from build123d import *

# Parameters (mm, degrees)
SKETCH1_W             = 278.511
SKETCH1_H             = 129.9972
BOSS_EXTRUDE1_DEPTH   = 4.191
F_2_56_TAPPED_HOLE2_D = 1.778
F_8_32_TAPPED_HOLE1_D = 3.4544
CUT_EXTRUDE1_REACH    = 309.384
SKETCH25_R            = 22.86
CUT_EXTRUDE2_REACH    = 309.384
SKETCH27_R            = 4.1656
SKETCH27_R_2          = 1.905


with BuildPart() as part:
    # Sketch1 → Boss-Extrude1 (new body)
    with BuildSketch(Plane(origin=(0, 0, 0), x_dir=(0, 0, -1), z_dir=(1, 0, 0))):
        with Locations((139.2555, 64.9986)):
            Rectangle(SKETCH1_W, SKETCH1_H)
    extrude(amount=BOSS_EXTRUDE1_DEPTH)

    # #2-56 Tapped Hole2 (through all)
    with Locations(Plane(origin=(4.191, 0, 0), x_dir=(0, 0, -1), z_dir=(1, 0, 0))):
        with Locations((38.1, 83.9724), (38.1, 110.9472), (60.452, 97.4598), (73.152, 110.9472), (73.152, 83.9724), (95.504, 97.4598)):
            Hole(F_2_56_TAPPED_HOLE2_D / 2)

    # #8-32 Tapped Hole1 (through all)
    with Locations(Plane(origin=(4.191, 0, 0), x_dir=(0, 0, -1), z_dir=(1, 0, 0))):
        with Locations((114.3, 60.9092), (114.3, 110.9472), (164.338, 110.9472), (164.338, 60.9092)):
            Hole(F_8_32_TAPPED_HOLE1_D / 2)

    # Sketch25 → Cut-Extrude1 (cut, up to next)
    with BuildSketch(Plane(origin=(4.191, 0, 0), x_dir=(0, 0, -1), z_dir=(1, 0, 0)), mode=Mode.PRIVATE) as cut_extrude1_sk1:
        with Locations((139.319, 85.9282)):
            Circle(SKETCH25_R)
    cut_extrude1_tool1 = extrude(cut_extrude1_sk1.sketch, amount=-CUT_EXTRUDE1_REACH, mode=Mode.PRIVATE) & part.part
    add(cut_extrude1_tool1.solids().sort_by_distance((4.191, 85.9282, -139.319))[0], mode=Mode.SUBTRACT)

    # Sketch27 → Cut-Extrude2 (cut, up to next)
    with BuildSketch(Plane(origin=(4.191, 0, 0), x_dir=(0, 0, -1), z_dir=(1, 0, 0)), mode=Mode.PRIVATE) as cut_extrude2_sk1:
        with Locations((221.361, 98.2472)):
            Circle(SKETCH27_R)
    cut_extrude2_tool1 = extrude(cut_extrude2_sk1.sketch, amount=-CUT_EXTRUDE2_REACH, mode=Mode.PRIVATE) & part.part
    # Sketch27 → Cut-Extrude2 (cut, up to next)
    with BuildSketch(Plane(origin=(4.191, 0, 0), x_dir=(0, 0, -1), z_dir=(1, 0, 0)), mode=Mode.PRIVATE) as cut_extrude2_sk2:
        with Locations((211.836, 98.2472)):
            Circle(SKETCH27_R_2)
    cut_extrude2_tool2 = extrude(cut_extrude2_sk2.sketch, amount=-CUT_EXTRUDE2_REACH, mode=Mode.PRIVATE) & part.part
    # Sketch27 → Cut-Extrude2 (cut, up to next)
    with BuildSketch(Plane(origin=(4.191, 0, 0), x_dir=(0, 0, -1), z_dir=(1, 0, 0)), mode=Mode.PRIVATE) as cut_extrude2_sk3:
        with Locations((230.886, 98.2472)):
            Circle(SKETCH27_R)
    cut_extrude2_tool3 = extrude(cut_extrude2_sk3.sketch, amount=-CUT_EXTRUDE2_REACH, mode=Mode.PRIVATE) & part.part
    # Sketch27 → Cut-Extrude2 (cut, up to next)
    with BuildSketch(Plane(origin=(4.191, 0, 0), x_dir=(0, 0, -1), z_dir=(1, 0, 0)), mode=Mode.PRIVATE) as cut_extrude2_sk4:
        with Locations((240.411, 98.2472)):
            Circle(SKETCH27_R_2)
    cut_extrude2_tool4 = extrude(cut_extrude2_sk4.sketch, amount=-CUT_EXTRUDE2_REACH, mode=Mode.PRIVATE) & part.part
    add(cut_extrude2_tool1.solids().sort_by_distance((4.191, 98.2472, -221.361))[0], mode=Mode.SUBTRACT)
    add(cut_extrude2_tool2.solids().sort_by_distance((4.191, 98.2472, -211.836))[0], mode=Mode.SUBTRACT)
    add(cut_extrude2_tool3.solids().sort_by_distance((4.191, 98.2472, -230.886))[0], mode=Mode.SUBTRACT)
    add(cut_extrude2_tool4.solids().sort_by_distance((4.191, 98.2472, -240.411))[0], mode=Mode.SUBTRACT)


solid = part.part
Could you check a few things on this model? Use its own coordinates, in mm. Round coordinates to 2 decimals unless told otherwise and drop trailing zeros. Loops run counter-clockwise (first coordinate to the right, second up) from the corner with the lowest first, then second, coordinate; pieces in that order, holes last. Notation, with made-up numbers: (25.5, 50.25) -> (47.5, 50.25) arc R37 cw to (47.5, 86.25) -> close; hole circle Ø7 at (46, 3.5). An arc over 180 degrees is marked (long way). Use CSV: the item, a comma, the result in double quotes.
(1) Suppose I cut it at A-A on y = 74. Write out the boundary of the cut face in (x, z).
Return value:
outline,"(0, -278.51) -> (4.19, -278.51) -> (4.19, -158.82) -> (0, -158.82) -> close; (0, -119.82) -> (4.19, -119.82) -> (4.19, 0) -> (0, 0) -> close"
(2) If I drill on probe 1 along Y at (x, z) = (0.9, -38.1); probe 2 along Z at (x, y) = (3.95, 111); probe 3 along Z at (x, y) = (1.55, 99), over which ranges is the centre line in solid material (lowest first)? Write a range as [from, to].
Return value:
probe 1,"y = [0, 83.08], [84.86, 110.06], [111.84, 130]"
probe 2,"z = [-278.51, -166.06], [-162.61, -116.03], [-112.57, -74.04], [-72.26, -38.99], [-37.21, 0]"
probe 3,"z = [-278.51, -242.16], [-238.66, -234.98], [-226.79, -225.46], [-217.26, -213.59], [-210.09, -158.07], [-120.57, 0]"
(3) Suppose I cut it at B-B on x = 0.8. Give the number of separate pieces and of enclosed holes in the cut face, plus the area to 3 significant figures.
Return value:
separate pieces,"1"
enclosed holes,"15"
area,"34,400 mm²"
(4) Will this pin go through, and if not, where does the flat tip stop? pin 1 Ø2.5 at (y, z) = (98.25, -240.41) entering from -X.
Return value:
pin 1,"passes through"
(5) If we mould it in two halves opening along Y, with no side actions, what happens to faces 1 (the flat face through (4.191, 51, -137)), 2 (the cylindrical face through (2.125, 101.76, -233.125))? For each: +Y half, -Y half, draft (parallel to the pull), parting line (faces both ways), or undercut.
Return value:
face 1,"draft"
face 2,"undercut"
